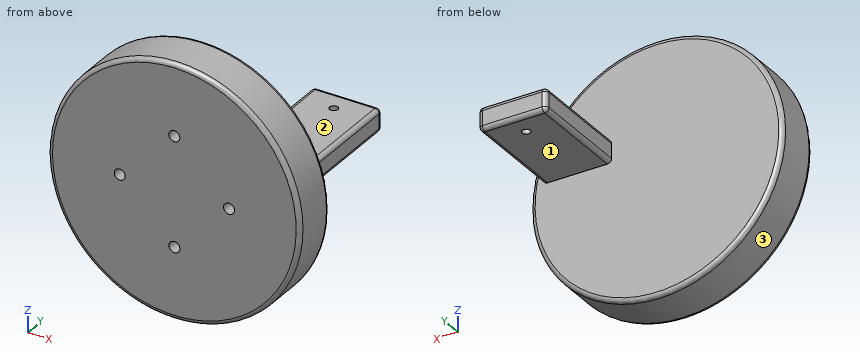
```python
from build123d import *

# Parameters (mm, degrees)
SKETCH_2_R          = 30
EXTRUDE_1_DEPTH     = 11
SKETCH_3_W          = 16.2
SKETCH_3_H          = 25
SKETCH_3_R          = 1
EXTRUDE_2_DEPTH     = 5.5
FILLET_1_R          = 1
SKETCH_4_R          = 1.3
CUT_EXTRUDE_1_DEPTH = 5


with BuildPart() as part:
    # 草图2 → 凸台-拉伸1 (new body)
    with BuildSketch(Plane(origin=(0, 0, 0), x_dir=(1, 0, 0), z_dir=(0, 1, 0))):
        with Locations(Location((0, 0, 0), (0, 0, 270))):
            Circle(SKETCH_2_R)
    extrude(amount=EXTRUDE_1_DEPTH)

    # 草图3 → 凸台-拉伸2 (add)
    with BuildSketch(Plane.XY.offset(4.63)):
        with Locations((18.9, 23.5)):
            Rectangle(SKETCH_3_W, SKETCH_3_H)
        with Locations((18.9, 30.67)):
            Circle(SKETCH_3_R, mode=Mode.SUBTRACT)
    extrude(amount=EXTRUDE_2_DEPTH)

    # 圆角1
    fillet_1_edges = [part.edges().sort_by_distance(p)[0] for p in [
        (27, 36, 7.38),
        (10.8, 23.5, 4.63),
        (10.8, 36, 7.38),
        (0, 0, -30),
        (0, 11, -30),
        (27, 23.5, 10.13),
        (18.9, 36, 10.13),
        (10.8, 23.5, 10.13),
        (27, 23.5, 4.63),
        (18.9, 36, 4.63),
    ]]
    fillet(fillet_1_edges, radius=FILLET_1_R)

    # 草图4 → 切除-拉伸1 (cut)
    with BuildSketch(Plane(origin=(0, 0, 0), x_dir=(-1, 0, 0), z_dir=(0, -1, 0))):
        with Locations(Location((0, -13, 0), (0, 0, 90))):
            Circle(SKETCH_4_R)
        with Locations(Location((-13, 0, 0), (0, 0, 90))):
            Circle(SKETCH_4_R)
        with Locations(Location((0, 13, 0), (0, 0, 90))):
            Circle(SKETCH_4_R)
        with Locations(Location((13, 0, 0), (0, 0, 90))):
            Circle(SKETCH_4_R)
    extrude(amount=-CUT_EXTRUDE_1_DEPTH, mode=Mode.SUBTRACT)


solid = part.part
```
Geometry: final body of the model. Coordinates: model frame, mm. Face numbers are marked on the shaded views. A direction names the side the tool comes from. Round coordinates to 2 decimals unless told otherwise and drop trailing zeros. Order: outer loops, then holes, each group sorted by start corner. A loop starts at its lowest first (then second) coordinate and runs counter-clockwise, first axis right, second up. Notation, with made-up numbers: M -8,65.25 L 33,65.25 A25 ccw 33,79.25 Z; hole C -21,73 d2. An arc over 180 degrees is marked long. Use one line per item in the form item = value. Start each with the question number.
Q1. Pin query (flat end, axial travel): pin 1 Ø1.7 at (y, z) = (18.5, 7) entering from +X; pin 2 Ø4 at (x, z) = (13.5, 20.5) entering from +Y; pin 3 Ø12 at (y, z) = (7.5, 20) entering from +X. Return the tip coordinate at first contact, or that it passes through.
Q2. Material intervals for line 1 (Y direction, x = 12, z = 2.5); line 2 (X direction, y = 2.5, z = -12); line 3 (Z direction, x = 1, y = 8), sorted ascending. Write a range as [from, to].
Q3. Access query for the marked faces 1, 2 and 3. Directions: +Z, -Z, +X, -X, +Y, -Y. A direction counts if a zero-diameter tool reaches every point of the face in a straight line with its end or side. Return the directions, or none.
Q4. Cut plane D-D (y = 9). Return loops of the section in (x, z), and give its area (3 significant figures).
Q5. Cut plane C-C (x = 0). Return loops of the section in (y, z), and give its area (3 significant figures).
Q6. Cut plane A-A (y = 21). Return loops of the section in (x, z).
Q7. Cut plane B-B (z = 0). Return loops of the section in (x, y).
Geometry results:
q1.pin_1 = 27
q1.pin_2 = 11
q1.pin_3 = 26.53
q2.line_1 = [0, 11]
q2.line_2 = [-27.5, -0.83], [0.83, 27.5]
q2.line_3 = [-29.98, 29.98]
q3.face_1 = -Z, +X, -X, +Y
q3.face_2 = +Z, +X, -X, +Y
q3.face_3 = +Y, -Y
q4.outline = C 0,0 d60
q4.area = 2,830 mm^2
q5.outline = M 0,-29 A1 ccw 1,-30 L 10,-30 A1 ccw 11,-29 L 11,29 A1 ccw 10,30 L 1,30 A1 ccw 0,29 L 0,14.3 L 5,14.3 L 5,11.7 L 0,11.7 L 0,-11.7 L 5,-11.7 L 5,-14.3 L 0,-14.3 Z
q5.area = 633 mm^2
q6.outline = M 10.8,5.63 A1 ccw 11.8,4.63 L 26,4.63 A1 ccw 27,5.63 L 27,9.13 A1 ccw 26,10.13 L 11.8,10.13 A1 ccw 10.8,9.13 Z
q7.outline = M -30,1 A1 ccw -29,0 L -14.3,0 L -14.3,5 L -11.7,5 L -11.7,0 L 11.7,0 L 11.7,5 L 14.3,5 L 14.3,0 L 29,0 A1 ccw 30,1 L 30,10 A1 ccw 29,11 L -29,11 A1 ccw -30,10 Z
